```python
from build123d import *

# Parameters (mm, degrees)
SKETCH1_W           = 152.4
SKETCH1_H           = 127
BOSS_EXTRUDE1_DEPTH = 4.7625
SKETCH2_R           = 2.794
CUT_EXTRUDE1_DEPTH  = 100.304437999
FILLET1_R           = 2.54
SKETCH4_W           = 15.599974926
SKETCH4_H           = 70.968900013
CUT_EXTRUDE2_DEPTH  = 100.304437999
SKETCH5_RX          = 35.484450006
SKETCH5_RY          = 14.605
CUT_EXTRUDE3_DEPTH  = 100.304437999


with BuildPart() as part:
    # Sketch1 → Boss-Extrude1 (new body)
    with BuildSketch(Plane(origin=(0, 0, 0), x_dir=(1, 0, 0), z_dir=(0, 1, 0))):
        Rectangle(SKETCH1_W, SKETCH1_H)
    extrude(amount=BOSS_EXTRUDE1_DEPTH)

    # Sketch2 → Cut-Extrude1 (cut, through all)
    with BuildSketch(Plane(origin=(0, 4.7625, 0), x_dir=(1, 0, 0), z_dir=(0, 1, 0))):
        with Locations(Location((71.794813785, -59.510435834, 0), (0, 0, 270))):
            Circle(SKETCH2_R)
        with Locations(Location((71.794813785, 59.510435834, 0), (0, 0, 270))):
            Circle(SKETCH2_R)
    cut_extrude1 = extrude(amount=-CUT_EXTRUDE1_DEPTH, mode=Mode.SUBTRACT)

    # Mirror1: Cut-Extrude1 across plane
    add(cut_extrude1.mirror(Plane(origin=(0, 0, 0), x_dir=(0, 0, 1), z_dir=(1, 0, 0))), mode=Mode.SUBTRACT)

    # Fillet1
    fillet1_edges = [part.edges().sort_by_distance(p)[0] for p in [
        (76.2, 2.38125, 63.5),
        (-76.2, 2.38125, 63.5),
        (-76.2, 2.38125, -63.5),
        (76.2, 2.38125, -63.5),
    ]]
    fillet(fillet1_edges, radius=FILLET1_R)

    # Sketch4 → Cut-Extrude2 (cut, through all)
    with BuildSketch(Plane(origin=(0, 4.7625, 0), x_dir=(1, 0, 0), z_dir=(0, 1, 0))):
        with Locations((-50.05790393, -1.440073651)):
            Rectangle(SKETCH4_W, SKETCH4_H)
    extrude(amount=-CUT_EXTRUDE2_DEPTH, mode=Mode.SUBTRACT)

    # Sketch5 → Cut-Extrude3 (cut, through all)
    with BuildSketch(Plane(origin=(0, 4.7625, 0), x_dir=(1, 0, 0), z_dir=(0, 1, 0))):
        with Locations(Location((-57.857891393, -1.44007365), (0, 0, -90))):
            Ellipse(SKETCH5_RX, SKETCH5_RY)
    extrude(amount=-CUT_EXTRUDE3_DEPTH, mode=Mode.SUBTRACT)


solid = part.part
```
Model file for the job. Use its own axes, mm. A direction names the side the tool comes from. Round coordinates to 2 decimals unless told otherwise and drop trailing zeros. One line per item, written item: value.
(1) Two-plate mould, pull along X, no slides. Class faces 3 (the cylindrical face through (-74.565, 2.415, 59.147)), 4 (the flat face through (-76.2, 2, 1)), 5 (the flat face through (-1, 2, -63.5)): pulls with the +X half, pulls with the -X half, needs draft (parallel to the pull), parting line crosses it, or undercut.
Values follow:
face 3: undercut
face 4: pulls with the -X half
face 5: needs draft
(2) Wall check: probe 1 along Z at (x, y) = (-42.5, 4.5); probe 2 along X at (y, z) = (3.2, 1); probe 3 along X at (y, z) = (3.6, 7). Give the ranges that are in metal, low to high.
Values follow:
probe 1: z = -63.5 to -34.04, 36.92 to 63.5
probe 2: x = -76.2 to -72.46, -42.26 to 76.2
probe 3: x = -76.2 to -72.28, -42.26 to 76.2
(3) Cut at A-A, the plane y = 3.05. Give the number of separate pieces and of enclosed holes in the cut face, plus the area to 3 significant figures.
Values follow:
separate pieces: 1
enclosed holes: 5
area: 17,300 mm²
(4) 3-axis set-ups, long thin cutter, end or side, ignore diameter. For faces 1 (the flat face through (-1, 0, -1)), 2 (the flat face through (-50, 2, 36.925)): which of +Z, -Z, +X, -X, +Y, -Y reach the whole face in a straight line?
Values follow:
face 1: +Z, -Z, +X, -X, -Y
face 2: +Y, -Y
